Check sheet for the drawn part. Datum: minimum x, y, z corner. Units: mm. A direction names the side the tool comes from. Round coordinates to 2 decimals unless told otherwise and drop trailing zeros. Write each loop counter-clockwise with the first axis right and the second up, starting at its lowest first coordinate (ties: lowest second). Pieces come first, ordered by that corner, then holes. Notation, with made-up numbers: (-8.5, -35.5) -> (30.5, -35.5) arc R37 ccw to (30.5, 2.5) -> close; hole circle Ø7 at (7, 36.25). An arc over 180 degrees is marked (long way). Use a Markdown table: item, result.
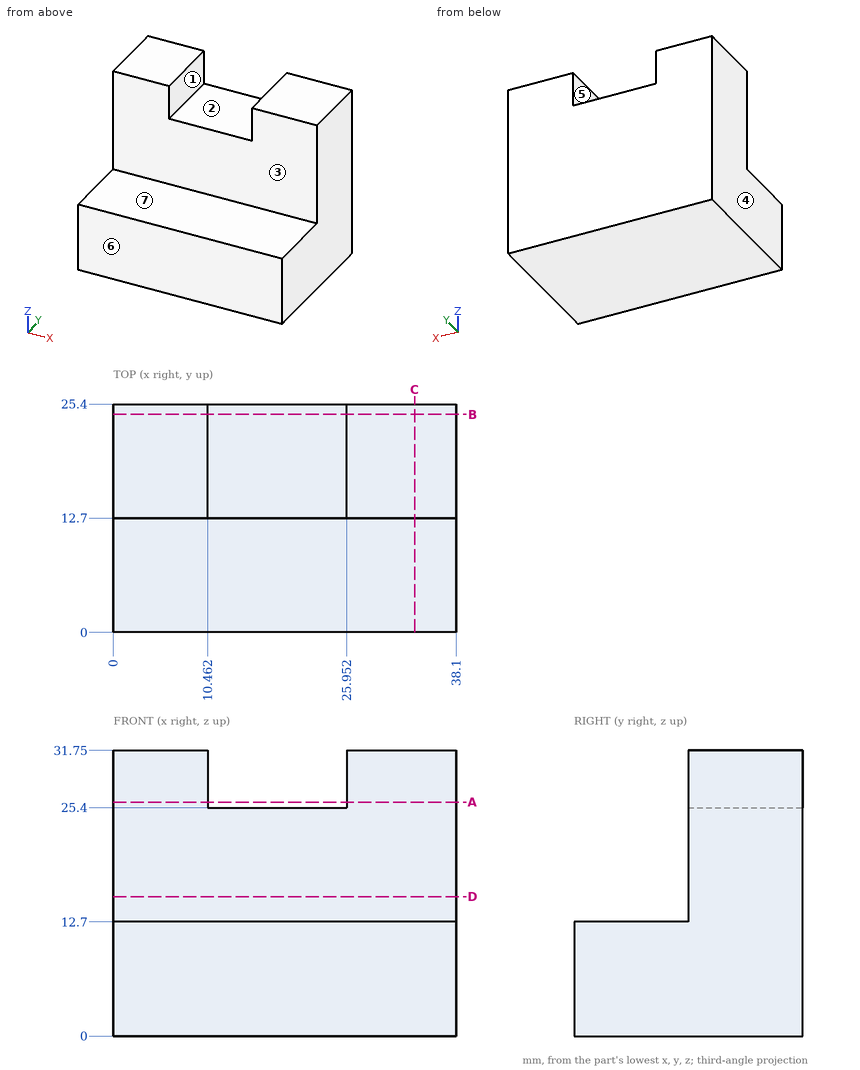
(1) Section check B-B on y = 24.25. Record the cut outline in (x, z).
A:
| item | result |
|---|---|
| outline | (0, 0) -> (38.1, 0) -> (38.1, 31.75) -> (25.95, 31.75) -> (25.95, 25.4) -> (10.46, 25.4) -> (10.46, 31.75) -> (0, 31.75) -> close |
(2) Access from +Z, -Z, +X, -X, +Y, -Y to the whole of each face (thin tool, end or side, straight path). Record for the marked faces 5, 6 and 7.
A:
| item | result |
|---|---|
| face 5 | +Z, +Y, -Y |
| face 6 | +Z, -Z, +X, -X, -Y |
| face 7 | +Z, +X, -X, -Y |
(3) Section check C-C on x = 33.5. Record the cut outline in (y, z).
A:
| item | result |
|---|---|
| outline | (0, 0) -> (25.4, 0) -> (25.4, 31.75) -> (12.7, 31.75) -> (12.7, 12.7) -> (0, 12.7) -> close |
(4) Section check A-A on z = 26. Record the cut outline in (x, y), plus the area to 3 significant figures.
A:
| item | result |
|---|---|
| outline | (0, 12.7) -> (10.46, 12.7) -> (10.46, 25.4) -> (0, 25.4) -> close; (25.95, 12.7) -> (38.1, 12.7) -> (38.1, 25.4) -> (25.95, 25.4) -> close |
| area | 287 mm2 |
(5) Release check for a two-part mould opening along X. For the marked faces 1, 2, 3 and 4 record: +X half, -X half, draft (parallel to the pull), parting line (faces both ways), or undercut.
A:
| item | result |
|---|---|
| face 1 | undercut |
| face 2 | undercut |
| face 3 | draft |
| face 4 | -X half |
(6) Thickness scan on line 1 (X direction, y = 18, z = 30.5); line 2 (Z direction, x = 20.5, y = 6.75); line 3 (Y direction, x = 5, z = 13.5). Record the ranges inside material, lowest first.
A:
| item | result |
|---|---|
| line 1 | x = 0 to 10.46, 25.95 to 38.1 |
| line 2 | z = 0 to 12.7 |
| line 3 | y = 12.7 to 25.4 |
(7) Gauge pin test, flat ends, axial feed: pin 1 Ø10 at (x, y) = (12, 3.5) entering from +Z; pin 2 Ø12 at (x, z) = (32, 19) entering from -Y. Record the tip position at first contact, or that the pin passes through.
A:
| item | result |
|---|---|
| pin 1 | stops at z = 12.7 |
| pin 2 | stops at y = 12.7 |
(8) Section check D-D on z = 15.5. Record the cut outline in (x, y).
A:
| item | result |
|---|---|
| outline | (0, 12.7) -> (38.1, 12.7) -> (38.1, 25.4) -> (0, 25.4) -> close |
